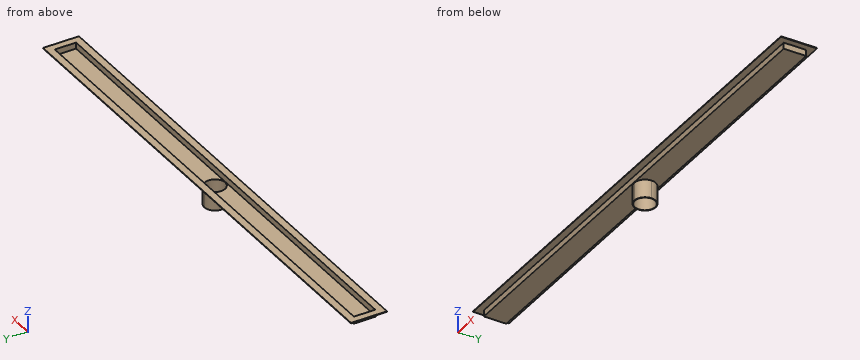
from build123d import *

# Parameters (mm, degrees)
F0_W     = 1406.525
F0_H     = 63.5
F0_W_2   = 1444.625
F0_H_2   = 101.6
F1_DEPTH = 1.5875
F0_R     = 28.575
F2_DEPTH = 19.05
F3_DEPTH = 69.85
F4_DEPTH = 17.4625
F5_DEPTH = 69.851


with BuildPart() as f1:
    # F0 (on Top) → F1 (new body)
    with BuildSketch(Plane.XY):
        with Locations((722.3125, 50.8)):
            Rectangle(F0_W, F0_H)
        Polygon((20.6375, 80.9625), (722.3125, 80.9625), (1423.9875, 80.9625), (1423.9875, 20.6375), (722.3125, 20.6375), (20.6375, 20.6375), align=None, mode=Mode.SUBTRACT)
        with Locations((722.3125, 50.8)):
            Rectangle(F0_W_2, F0_H_2)
        with Locations((722.3125, 50.8)):
            Rectangle(F0_W, F0_H, mode=Mode.SUBTRACT)
    extrude(amount=-F1_DEPTH)

    # F0 (on Top) → F2 (join)
    with BuildSketch(Plane.XY):
        with Locations((722.3125, 50.8)):
            Rectangle(F0_W, F0_H)
        Polygon((20.6375, 80.9625), (722.3125, 80.9625), (1423.9875, 80.9625), (1423.9875, 20.6375), (722.3125, 20.6375), (20.6375, 20.6375), align=None, mode=Mode.SUBTRACT)
        with BuildLine():
            ThreePointArc((722.3125, 20.6375), (692.15, 50.8), (722.3125, 80.9625))
            Line((722.3125, 80.9625), (20.6375, 80.9625))
            Line((20.6375, 80.9625), (20.6375, 20.6375))
            Line((20.6375, 20.6375), (722.3125, 20.6375))
        make_face()
        with BuildLine():
            ThreePointArc((722.3125, 80.9625), (743.640608, 72.128108), (752.475, 50.8))
            ThreePointArc((752.475, 50.8), (743.640608, 29.471892), (722.3125, 20.6375))
            Line((722.3125, 20.6375), (1423.9875, 20.6375))
            Line((1423.9875, 20.6375), (1423.9875, 80.9625))
            Line((1423.9875, 80.9625), (722.3125, 80.9625))
        make_face()
        with BuildLine():
            ThreePointArc((722.3125, 20.6375), (743.640608, 29.471892), (752.475, 50.8))
            ThreePointArc((752.475, 50.8), (743.640608, 72.128108), (722.3125, 80.9625))
            ThreePointArc((722.3125, 80.9625), (692.15, 50.8), (722.3125, 20.6375))
        make_face()
        with Locations((722.3125, 50.8)):
            Circle(F0_R, mode=Mode.SUBTRACT)
        with Locations((722.3125, 50.8)):
            Circle(F0_R)
    extrude(amount=-F2_DEPTH)

    # F0 (on Top) → F3 (join)
    with BuildSketch(Plane.XY):
        with BuildLine():
            ThreePointArc((722.3125, 20.6375), (743.640608, 29.471892), (752.475, 50.8))
            ThreePointArc((752.475, 50.8), (743.640608, 72.128108), (722.3125, 80.9625))
            ThreePointArc((722.3125, 80.9625), (692.15, 50.8), (722.3125, 20.6375))
        make_face()
        with Locations((722.3125, 50.8)):
            Circle(F0_R, mode=Mode.SUBTRACT)
    extrude(amount=-F3_DEPTH)

    # F0 (on Top) → F4 (cut)
    with BuildSketch(Plane.XY):
        with BuildLine():
            ThreePointArc((722.3125, 20.6375), (692.15, 50.8), (722.3125, 80.9625))
            Line((722.3125, 80.9625), (20.6375, 80.9625))
            Line((20.6375, 80.9625), (20.6375, 20.6375))
            Line((20.6375, 20.6375), (722.3125, 20.6375))
        make_face()
        with BuildLine():
            ThreePointArc((722.3125, 80.9625), (743.640608, 72.128108), (752.475, 50.8))
            ThreePointArc((752.475, 50.8), (743.640608, 29.471892), (722.3125, 20.6375))
            Line((722.3125, 20.6375), (1423.9875, 20.6375))
            Line((1423.9875, 20.6375), (1423.9875, 80.9625))
            Line((1423.9875, 80.9625), (722.3125, 80.9625))
        make_face()
        with BuildLine():
            ThreePointArc((722.3125, 20.6375), (743.640608, 29.471892), (752.475, 50.8))
            ThreePointArc((752.475, 50.8), (743.640608, 72.128108), (722.3125, 80.9625))
            ThreePointArc((722.3125, 80.9625), (692.15, 50.8), (722.3125, 20.6375))
        make_face()
        with Locations((722.3125, 50.8)):
            Circle(F0_R, mode=Mode.SUBTRACT)
        with Locations((722.3125, 50.8)):
            Circle(F0_R)
    extrude(amount=-F4_DEPTH, mode=Mode.SUBTRACT)

    # F0 (on Top) → F5 (cut, through all)
    with BuildSketch(Plane.XY):
        with Locations((722.3125, 50.8)):
            Circle(F0_R)
    extrude(amount=-F5_DEPTH, mode=Mode.SUBTRACT)


solid = f1.part
For this review, take the finished solid that the model builds, in its own axes (mm). Round coordinates to 2 decimals unless told otherwise and drop trailing zeros. Order: outer loops, then holes, each group sorted by start corner. A loop starts at its lowest first (then second) coordinate and runs counter-clockwise, first axis right, second up. Notation, with made-up numbers: M -15.75,16.25 L 41.25,16.25 A26 ccw 41.25,35.25 Z; hole C 53.25,-2 d8. An arc over 180 degrees is marked long. Use a Markdown table: item, result. Add a question column.
Item 1: Insertion check: pin 1 (5 mm diameter, centred on x = 596, z = -9.5, fed in from +Y); pin 2 (19 mm diameter, centred on x = 710, y = 60.5, fed in from -Z); pin 3 (4 mm diameter, centred on y = 26.5, z = -10, fed in from -X); pin 4 (19 mm diameter, centred on y = 61.5, z = -6.5, fed in from -X). Each pin has a flat end and moves straight along its axis. Give the tip position at first contact, or say it passes through.
Item 2: Add section A-A, the plane x = 796. Give the boundary of the cut face in (y, z).
Item 3: To check wall thickness, follow line 1 along X through (y, z) = (50, -49); line 2 along Y through (x, z) = (131, -8.5); line 3 along Z through (x, y) = (498.5, 17). State the ranges of each line that lie inside material, in increasing order.
Geometry results:
| question | item | result |
|---|---|---|
| 1 | pin 1 | stops at y = 82.55 |
| 1 | pin 2 | passes through |
| 1 | pin 3 | stops at x = 19.05 |
| 1 | pin 4 | stops at x = 0 |
| 2 | outline | M 0,-1.59 L 19.05,-1.59 L 19.05,-19.05 L 82.55,-19.05 L 82.55,-1.59 L 101.6,-1.59 L 101.6,0 L 80.96,0 L 80.96,-17.46 L 20.64,-17.46 L 20.64,0 L 0,0 Z |
| 3 | line 1 | x = 692.16 to 693.75, 750.88 to 752.46 |
| 3 | line 2 | y = 19.05 to 20.64, 80.96 to 82.55 |
| 3 | line 3 | z = -1.59 to 0 |
